Here's how the part is built. I have some questions about the finished solid (model axes, mm). Coordinates: 2 decimals unless noted, no trailing zeros. Write each loop counter-clockwise with the first axis right and the second up, starting at its lowest first coordinate (ties: lowest second). Pieces come first, ordered by that corner, then holes. Notation, with made-up numbers: (68, -28.75) -> (101, -28.75) arc R32 ccw to (101, 1.25) -> close; hole circle Ø11 at (-35, 84). An arc over 180 degrees is marked (long way). Answer in a Markdown table with one row per item. Add a question column.
from build123d import *

# Parameters (mm, degrees)
ESQUISSE1_W             = 80
ESQUISSE1_H             = 50
BOSS_EXTRU_1_DEPTH      = 8
ESQUISSE2_R             = 3.5
ENL_V_MAT_EXTRU_1_DEPTH = 17


with BuildPart() as part:
    # Esquisse1 → Boss.-Extru.1 (new body, symmetric)
    with BuildSketch(Plane.XY):
        Rectangle(ESQUISSE1_W, ESQUISSE1_H)
    extrude(amount=BOSS_EXTRU_1_DEPTH, both=True)

    # Esquisse2 → Enlèv. mat.-Extru.1 (cut, through all)
    with BuildSketch(Plane.XY.offset(8)):
        with Locations((-30, 17.5)):
            Circle(ESQUISSE2_R)
        with Locations(Location((30, 17.5, 0), (0, 0, 180))):  # turned: the seam where the file's is
            Circle(ESQUISSE2_R)
        with Locations((-30, -17.5)):
            Circle(ESQUISSE2_R)
        with Locations((30, -17.5)):
            Circle(ESQUISSE2_R)
    extrude(amount=-ENL_V_MAT_EXTRU_1_DEPTH, mode=Mode.SUBTRACT)


solid = part.part
Q1. If we mould it in two halves opening along Y, with no side actions, what happens to faces 1 (the cylindrical face through (26.66, 16.45, 0.11)), 2 (the flat face through (-40, 0, 0)), 3 (the flat face through (-1, -25, 0))? For each: pulls with the +Y half, pulls with the -Y half, needs draft (parallel to the pull), parting line crosses it, or undercut.
Q2. Imagine slicing it at B-B on y = 17.5. Please give me the cut outline in (x, z).
Q3. I'm going to push flat-ended pins straight in: P1, Ø5.5, axis at x = -30, y = -17.5, coming from the +Z side; P2, Ø9, axis at x = 30, y = 17.5, coming from the -Z side. Where does each tip first touch, or does it pass through?
Q4. Imagine slicing it at A-A on x = -30. Please give me the cut outline in (y, z).
Q5. Imagine slicing it at C-C on z = -6.25. Please give me the cut outline in (x, y).
Q6. I need wall thicknesses on line 1 (Y direction, x = 30, z = 2); line 2 (X direction, y = 16, z = 6); line 3 (Y direction, x = 28, z = -4.5). Which ranges of each line are inside material? Lowest first, please. Write a range as [from, to].
Result sheet:
| question | item | result |
|---|---|---|
| 1 | face 1 | undercut |
| 1 | face 2 | needs draft |
| 1 | face 3 | pulls with the -Y half |
| 2 | outline | (-40, -8) -> (-33.5, -8) -> (-33.5, 8) -> (-40, 8) -> close; (-26.5, -8) -> (26.5, -8) -> (26.5, 8) -> (-26.5, 8) -> close; (33.5, -8) -> (40, -8) -> (40, 8) -> (33.5, 8) -> close |
| 3 | P1 | passes through |
| 3 | P2 | stops at z = -8 |
| 4 | outline | (-25, -8) -> (-21, -8) -> (-21, 8) -> (-25, 8) -> close; (-14, -8) -> (14, -8) -> (14, 8) -> (-14, 8) -> close; (21, -8) -> (25, -8) -> (25, 8) -> (21, 8) -> close |
| 5 | outline | (-40, -25) -> (40, -25) -> (40, 25) -> (-40, 25) -> close; hole circle Ø7 at (-30, -17.5); hole circle Ø7 at (-30, 17.5); hole circle Ø7 at (30, -17.5); hole circle Ø7 at (30, 17.5) |
| 6 | line 1 | y = [-25, -21], [-14, 14], [21, 25] |
| 6 | line 2 | x = [-40, -33.16], [-26.84, 26.84], [33.16, 40] |
| 6 | line 3 | y = [-25, -20.37], [-14.63, 14.63], [20.37, 25] |
